```python
from build123d import *

# Parameters (mm, degrees)
F0_R     = 1.778
F1_DEPTH = 2.54
F2_R     = 5.08
F3_R     = 1.016


# Not quite as in the source:
# - a feature names something its author has since deleted; it is built from what else it names


with BuildPart() as f1:
    # F0 (on Front) → F1 (new body)
    with BuildSketch(Plane.XZ):
        with BuildLine():
            Line((0.762, 12.192), (-0.762, 12.192))
            Line((-0.762, 12.192), (-1.651, 9.652))
            Line((-1.651, 9.652), (-1.905, 7.3780332745))
            ThreePointArc((-1.905, 7.3780332745), (0, 7.8729912016), (1.905, 7.3780332745))
            Line((1.905, 7.3780332745), (1.651, 9.652))
            Line((1.651, 9.652), (0.762, 12.192))
        make_face()
        with BuildLine():
            ThreePointArc((1.905, 7.3780332745), (0, 7.8729912016), (-1.905, 7.3780332745))
            ThreePointArc((-1.905, 7.3780332745), (-2.3002813477, 7.1255844849), (-2.6625230681, 6.8276605496))
            ThreePointArc((-2.6625230681, 6.8276605496), (-3.7219334042, 5.168848297), (-3.8398778167, 3.2041352225))
            ThreePointArc((-3.8398778167, 3.2041352225), (-3.7219334042, 2.7501893548), (-3.5505297519, 2.3136134471))
            ThreePointArc((-3.5505297519, 2.3136134471), (-2.3002813477, 0.793453167), (-0.4681750033, 0.0741516359))
            ThreePointArc((-0.4681750033, 0.0741516359), (0, 0.0460464502), (0.4681750033, 0.0741516359))
            ThreePointArc((0.4681750033, 0.0741516359), (2.3002813477, 0.793453167), (3.5505297519, 2.3136134471))
            ThreePointArc((3.5505297519, 2.3136134471), (3.7219334042, 2.7501893548), (3.8398778167, 3.2041352225))
            ThreePointArc((3.8398778167, 3.2041352225), (3.8950302821, 3.5800387384), (3.9134723757, 3.9595188259))
            ThreePointArc((3.9134723757, 3.9595188259), (3.5871281349, 5.5240563868), (2.6625230681, 6.8276605496))
            ThreePointArc((2.6625230681, 6.8276605496), (2.3002813477, 7.1255844849), (1.905, 7.3780332745))
        make_face()
        with Locations((0, 3.9595188259)):
            Circle(F0_R, mode=Mode.SUBTRACT)
        with BuildLine():
            ThreePointArc((-3.8398778167, 3.2041352225), (-3.7219334042, 5.168848297), (-2.6625230681, 6.8276605496))
            Line((-2.6625230681, 6.8276605496), (-4.9036842568, 7.2887865573))
            Line((-4.9036842568, 7.2887865573), (-7.5940839162, 7.22820048))
            Line((-7.5940839162, 7.22820048), (-8.0650258156, 5.7787903492))
            Line((-8.0650258156, 5.7787903492), (-5.9240583722, 4.1483979405))
            Line((-5.9240583722, 4.1483979405), (-3.8398778167, 3.2041352225))
        make_face()
        with BuildLine():
            Line((4.9036842568, 7.2887865573), (2.6625230681, 6.8276605496))
            ThreePointArc((2.6625230681, 6.8276605496), (3.5871281349, 5.5240563868), (3.9134723757, 3.9595188259))
            ThreePointArc((3.9134723757, 3.9595188259), (3.8950302821, 3.5800387384), (3.8398778167, 3.2041352225))
            Line((3.8398778167, 3.2041352225), (5.9240583722, 4.1483979405))
            Line((5.9240583722, 4.1483979405), (8.0650258156, 5.7787903492))
            Line((8.0650258156, 5.7787903492), (7.5940839162, 7.22820048))
            Line((7.5940839162, 7.22820048), (4.9036842568, 7.2887865573))
        make_face()
        with BuildLine():
            ThreePointArc((-0.4681750033, 0.0741516359), (-2.3002813477, 0.793453167), (-3.5505297519, 2.3136134471))
            Line((-3.5505297519, 2.3136134471), (-4.6816435408, 0.3246382675))
            Line((-4.6816435408, 0.3246382675), (-5.4554019736, -2.2528059875))
            Line((-5.4554019736, -2.2528059875), (-4.2224600742, -3.148590712))
            Line((-4.2224600742, -3.148590712), (-2.0102694254, -1.6162286356))
            Line((-2.0102694254, -1.6162286356), (-0.4681750033, 0.0741516359))
        make_face()
        with BuildLine():
            Line((4.6816435408, 0.3246382675), (3.5505297519, 2.3136134471))
            ThreePointArc((3.5505297519, 2.3136134471), (2.3002813477, 0.793453167), (0.4681750033, 0.0741516359))
            Line((0.4681750033, 0.0741516359), (2.0102694254, -1.6162286356))
            Line((2.0102694254, -1.6162286356), (4.2224600742, -3.148590712))
            Line((4.2224600742, -3.148590712), (5.4554019736, -2.2528059875))
            Line((5.4554019736, -2.2528059875), (4.6816435408, 0.3246382675))
        make_face()
    extrude(amount=F1_DEPTH)

    # F2
    f2_edges = [f1.edges().sort_by_distance(p)[0] for p in [
        (1.651, -1.27, 9.652),
        (-4.903684, -1.27, 7.288787),
        (-4.681644, -1.27, 0.324638),
        (2.010269, -1.27, -1.616229),
        (5.924058, -1.27, 4.148398),
        (-1.651, -1.27, 9.652),
        (-5.924058, -1.27, 4.148398),
        (-2.010269, -1.27, -1.616229),
        (4.681644, -1.27, 0.324638),
        (4.903684, -1.27, 7.288787),
    ]]
    fillet(f2_edges, radius=F2_R)

    # F3
    f3_edges = [f1.edges().sort_by_distance(p)[0] for p in [
        (0.762, -1.27, 12.192),
        (-0.762, -1.27, 12.192),
        (-7.594084, -1.27, 7.2282),
        (-8.065026, -1.27, 5.77879),
        (-5.455402, -1.27, -2.252806),
        (-4.22246, -1.27, -3.148591),
        (4.22246, -1.27, -3.148591),
        (5.455402, -1.27, -2.252806),
        (8.065026, -1.27, 5.77879),
        (7.594084, -1.27, 7.2282),
    ]]
    fillet(f3_edges, radius=F3_R)


solid = f1.part
```
Verification items for the finished model (mm, model axes). A direction names the side the tool comes from. Coordinates: 2 decimals unless noted, no trailing zeros. Write each loop counter-clockwise with the first axis right and the second up, starting at its lowest first coordinate (ties: lowest second). Pieces come first, ordered by that corner, then holes. Notation, with made-up numbers: M 27,80.5 L 79,80.5 A20 cw 79,98.5 Z; hole C 63,89 d7. An arc over 180 degrees is marked long. Answer as a JSON object with one key per item and string values. Group by question number.
(1) Material ranges on line 1 (X direction, y = -0.8, z = 11.5); line 2 (X direction, y = -0.3, z = -2); line 3 (Z direction, x = 0.5, y = -0.3), recorded low to high.
(2) Cross-section at A-A, the plane x = -0.25. Record the cut outline in (y, z), and give its area (3 significant figures).
(3) Tool access check on faces 4 (the face through (2.03, -1.29, -1.59)), 5 (the face through (-3.5, -1.3, 7)), 6 (the face through (4.609, -1.252, 3.553)), 7 (the face through (-3.97, -1.25, 1.58)). Record the directions out of +Z, -Z, +X, -X, +Y, -Y that give a thin tool (end or side, any length) a straight path to the whole face; none if there is none.
(4) Gauge pin test, flat ends, axial feed: pin 1 (1 mm diameter, centred on x = 1.5, y = -1, fed in from -Z); pin 2 (1 mm diameter, centred on y = -2, z = 1, fed in from -X). Record the tip position at first contact, or that the pin passes through.
(5) Cross-section at C-C, the plane x = 7.25. Record the cut outline in (y, z).
(6) Cross-section at B-B, the plane z = 1.25. Record the cut outline in (x, y), and give its area (3 significant figures).
(7) Release check for a two-part mould opening along Z. For faces 1 (the face through (7.85, -1.29, 5.86)), 2 (the face through (3, -1.3, -2.3)), 3 (the face through (-3.724, -1.252, 2.756)) record: +Z half, -Z half, draft (parallel to the pull), parting line (faces both ways), or undercut.
Reply:
{
 "1": {"line 1": "-1 to 1", "line 2": "-5.28 to -2.56, 2.56 to 5.28", "line 3": "0.04 to 2.25, 5.67 to 12.08"},
 "2": {"outline": "M -2.54,0.05 L 0,0.05 L 0,2.2 L -2.54,2.2 Z; M -2.54,5.72 L 0,5.72 L 0,12.17 L -2.54,12.17 Z", "area": "21.8 mm²"},
 "3": {"face 4": "-Z, +Y, -Y", "face 5": "+Z, +Y, -Y", "face 6": "+X, +Y, -Y", "face 7": "-X, +Y, -Y"},
 "4": {"pin 1": "z = -1.56", "pin 2": "x = -4.57"},
 "5": {"outline": "M -2.54,5.16 L 0,5.16 L 0,7.16 L -2.54,7.16 Z"},
 "6": {"outline": "M -4.16,-2.54 L 4.16,-2.54 L 4.16,0 L -4.16,0 Z", "area": "21.1 mm²"},
 "7": {"face 1": "parting line", "face 2": "-Z half", "face 3": "undercut"}
}
